Input: part model. Units: mm. Frame: model coordinates. Face numbers are marked on the shaded views. A direction names the side the tool comes from. Round coordinates to 2 decimals unless told otherwise and drop trailing zeros. Loops run counter-clockwise (first coordinate to the right, second up) from the corner with the lowest first, then second, coordinate; pieces in that order, holes last.
(1) Draft query along X for the marked faces 3 and 4. Return one class per face: released by +X, released by -X, zero draft, split by the parting line, or undercut.
(2) Cut plane C-C, the plane y = -5. Output: boundary loops of the cut face in (x, z), and give its area (3 significant figures).
(3) Cut plane A-A, the plane x = 0. Output: boundary loops of the cut face in (y, z).
(4) Line query: line 1 (Z direction, x = -0.5, y = -23); line 2 (Y direction, x = 0, z = 85); line 3 (Z direction, x = 0, y = -14.5). Output: solid intervals per line, ascending.
(5) Access query for the marked faces 1 and 2. Directions: +Z, -Z, +X, -X, +Y, -Y. A direction counts if a zero-diameter tool reaches every point of the face in a straight line with its end or side. Return the directions, or none.
(6) Cut plane B-B, the plane z = 66.5. Output: boundary loops of the cut face in (x, y).
(7) First-contact query: pin 1 Ø2 at (x, z) = (-2.5, 83.5) entering from -Y; pin 2 Ø1 at (x, y) = (0.5, -48.5) entering from -Z; pin 3 Ø5 at (x, z) = (5, 57) entering from +Y. Flat tips, straight axial feed; report the tip coordinate or a pass-through.
from build123d import *

# Parameters (mm, degrees)
SKETCH1_R   = 6.35
SKETCH1_R_2 = 5.969


with BuildPart() as part:
    # Sweep1: sweep along a path in Sketch2
    with BuildLine(Plane(origin=(0, 0, 0), x_dir=(0, 0, -1), z_dir=(1, 0, 0))) as sweep1_path:
        Line((0, 0), (0, -31.75))
        ThreePointArc((0, -31.75), (-11.159231637, -58.690768363), (-38.1, -69.85))
        Line((-38.1, -69.85), (-139.7, -69.85))
    # Sketch1 → Sweep1 (sweep)
    with BuildSketch(Plane(origin=(0, 0, 0), x_dir=(1, 0, 0), z_dir=(0, 1, 0))):
        Circle(SKETCH1_R)
        Circle(SKETCH1_R_2, mode=Mode.SUBTRACT)
    sweep(path=sweep1_path.line)


solid = part.part
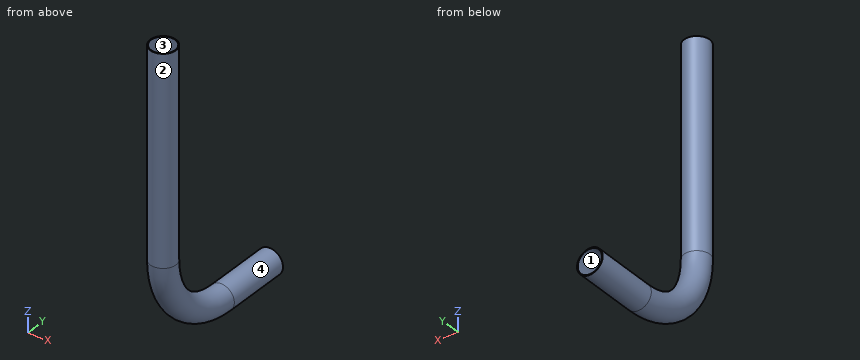
Reported:
1. face 3: undercut
1. face 4: split by the parting line
2. outline: circle Ø12.7 at (0, 0); hole circle Ø11.94 at (0, 0)
2. area: 14.7 mm2
3. outline: (-76.2, 38.1) arc R44.45 ccw to (-31.75, -6.35) - (0, -6.35) - (0, -5.97) - (-31.75, -5.97) arc R44.07 cw to (-75.82, 38.1) - (-75.82, 139.7) - (-76.2, 139.7) - close; (-63.88, 38.1) arc R32.13 ccw to (-31.75, 5.97) - (0, 5.97) - (0, 6.35) - (-31.75, 6.35) arc R31.75 cw to (-63.5, 38.1) - (-63.5, 139.7) - (-63.88, 139.7) - close
4. line 1: z = -6.33 to -5.95, 5.95 to 6.33
4. line 2: y = -76.2 to -75.82, -63.88 to -63.5
4. line 3: z = -6.35 to -5.97, 5.97 to 6.35
5. face 1: +Y
5. face 2: +Z
6. outline: circle Ø12.7 at (0, -69.85); hole circle Ø11.94 at (0, -69.85)
7. pin 1: stops at y = -76.02
7. pin 2: stops at z = -3.26
7. pin 3: stops at y = -64.01
